For this review, take the finished solid that the model builds, in its own axes (mm). Round coordinates to 2 decimals unless told otherwise and drop trailing zeros. Write each loop counter-clockwise with the first axis right and the second up, starting at its lowest first coordinate (ties: lowest second). Pieces come first, ordered by that corner, then holes.
from build123d import *

# Parameters (mm, degrees)
F0_R     = 25
F1_DEPTH = 4


with BuildPart() as f1:
    # F0 (on Top) → F1 (new body)
    with BuildSketch(Plane.XY):
        with BuildLine():
            Line((-94.75, -32.5), (94.75, -32.5))
            ThreePointArc((94.75, -32.5), (99.522971, -30.522971), (101.5, -25.75))
            Line((101.5, -25.75), (101.5, 25.75))
            ThreePointArc((101.5, 25.75), (99.522971, 30.522971), (94.75, 32.5))
            Line((94.75, 32.5), (-94.75, 32.5))
            ThreePointArc((-94.75, 32.5), (-99.522971, 30.522971), (-101.5, 25.75))
            Line((-101.5, 25.75), (-101.5, -25.75))
            ThreePointArc((-101.5, -25.75), (-99.522971, -30.522971), (-94.75, -32.5))
        make_face()
        with Locations((-68.25, 0)):
            Circle(F0_R, mode=Mode.SUBTRACT)
        with BuildLine():
            ThreePointArc((16, 19), (35, 0), (16, -19))
            Line((16, -19), (-16, -19))
            ThreePointArc((-16, -19), (-35, 0), (-16, 19))
            Line((-16, 19), (16, 19))
        make_face(mode=Mode.SUBTRACT)
        with Locations((68.25, 0)):
            Circle(F0_R, mode=Mode.SUBTRACT)
    extrude(amount=F1_DEPTH)


solid = f1.part
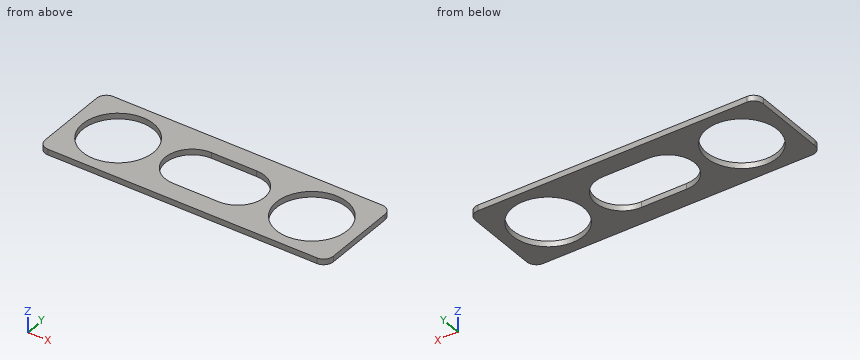
(1) For pin 1 Ø12 at (x, y) = (61, 13) entering from -Z, flat-tipped, find the tip position at first contact; note if it passes through.
Geometry check:
pin 1: passes through
(2) We need section C-C, the plane z = 2.4. Give the boundary of the cut face in (x, y), and give its area (3 significant figures).
Geometry check:
outline: (-101.5, -25.75) arc R6.75 ccw to (-94.75, -32.5) - (94.75, -32.5) arc R6.75 ccw to (101.5, -25.75) - (101.5, 25.75) arc R6.75 ccw to (94.75, 32.5) - (-94.75, 32.5) arc R6.75 ccw to (-101.5, 25.75) - close; hole circle Ø50 at (-68.25, 0); hole (-16, -19) - (16, -19) arc R19 ccw to (16, 19) - (-16, 19) arc R19 ccw to start; hole circle Ø50 at (68.25, 0)
area: 6,880 mm2
(3) For line 1 along Y through (x, z) = (-8, 1.8); line 2 along Y through (x, z) = (-68.25, 0.85); line 3 along X through (y, z) = (6, 0.9), list the stretches that pass through material, from the lowest coordinate up.
Geometry check:
line 1: y = -32.5 to -19, 19 to 32.5
line 2: y = -32.5 to -25, 25 to 32.5
line 3: x = -101.5 to -92.52, -43.98 to -34.03, 34.03 to 43.98, 92.52 to 101.5
(4) We need section B-B, the plane y = -2.5. Give the boundary of the cut face in (x, z), and give its area (3 significant figures).
Geometry check:
outline: (-101.5, 0) - (-93.12, 0) - (-93.12, 4) - (-101.5, 4) - close; (-43.38, 0) - (-34.83, 0) - (-34.83, 4) - (-43.38, 4) - close; (34.83, 0) - (43.38, 0) - (43.38, 4) - (34.83, 4) - close; (93.12, 0) - (101.5, 0) - (101.5, 4) - (93.12, 4) - close
area: 135 mm2
(5) We need section D-D, the plane x = -24. Give the boundary of the cut face in (y, z).
Geometry check:
outline: (-32.5, 0) - (-17.23, 0) - (-17.23, 4) - (-32.5, 4) - close; (17.23, 0) - (32.5, 0) - (32.5, 4) - (17.23, 4) - close
(6) We need section A-A, the plane x = -68.25. Give the boundary of the cut face in (y, z), and give its area (3 significant figures).
Geometry check:
outline: (-32.5, 0) - (-25, 0) - (-25, 4) - (-32.5, 4) - close; (25, 0) - (32.5, 0) - (32.5, 4) - (25, 4) - close
area: 60.0 mm2
